Design review of the part shown in the three views and the two pictorial views. Dimensions are in mm from the part's minimum x, y and z. Round coordinates to 2 decimals unless told otherwise and drop trailing zeros. Loops run counter-clockwise (first coordinate to the right, second up) from the corner with the lowest first, then second, coordinate; pieces in that order, holes last.
1) Take a section at A-A (y = 63.5). State the section outline as (x, z) points.
2) Wall thickness on L1, parallel to Y at x = 96.5, z = 2.8; L2, parallel to X at y = 50.5, z = 1.4: over which ranges is each line inside the solid? List them lowest first.
3) Insertion check: pin 1 (8 mm diameter, centred on x = 155, y = 130.5, fed in from -Z). The pin has a flat end and moves straight along its axis. Give the tip position at first contact, or say it passes through.
4) Take a section at B-B (x = 97). State the section outline as (y, z) points.
5) Take a section at C-C (z = 1.5). Give the number of separate pieces and of enclosed holes in the cut face, then the cut area to 3 significant figures.
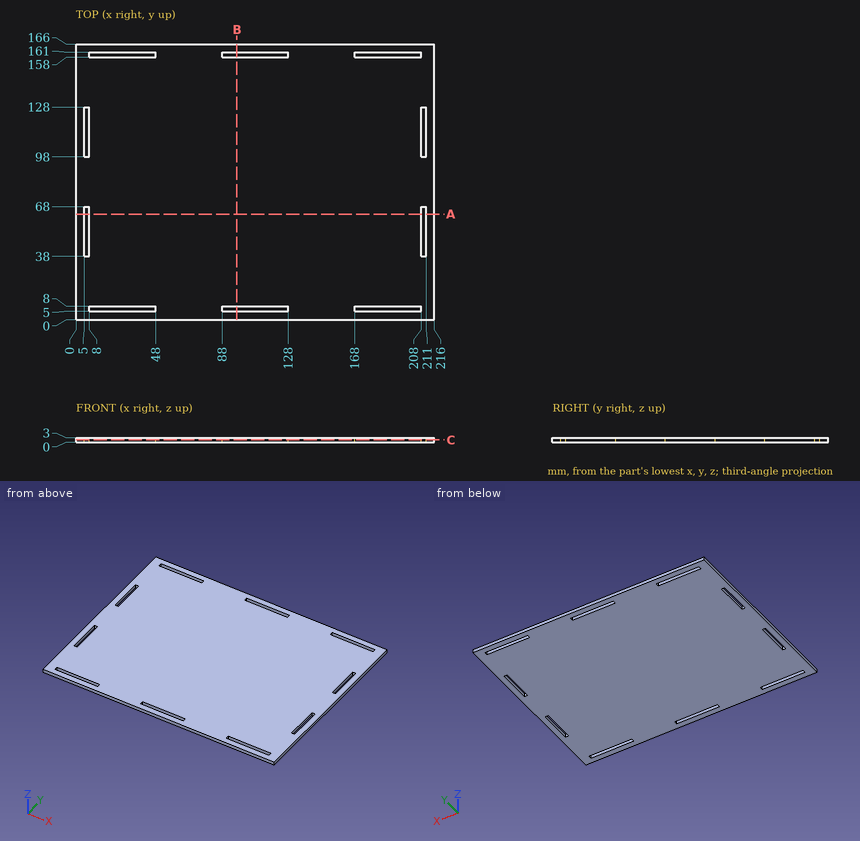
Response:
1. outline: (0, 0) - (5, 0) - (5, 3) - (0, 3) - close; (8, 0) - (208, 0) - (208, 3) - (8, 3) - close; (211, 0) - (216, 0) - (216, 3) - (211, 3) - close
2. L1: y = 0 to 5, 8 to 158, 161 to 166
2. L2: x = 0 to 5, 8 to 208, 211 to 216
3. pin 1: stops at z = 0
4. outline: (0, 0) - (5, 0) - (5, 3) - (0, 3) - close; (8, 0) - (158, 0) - (158, 3) - (8, 3) - close; (161, 0) - (166, 0) - (166, 3) - (161, 3) - close
5. separate pieces: 1
5. enclosed holes: 10
5. area: 34,800 mm2
